Part model, mm, in its own coordinate system. Face numbers are marked on the shaded views. A direction names the side the tool comes from. Round coordinates to 2 decimals unless told otherwise and drop trailing zeros. Write each question's results on one line, items separated by ' | '. Start each with the question number.
1. Drop flat-ended pins along their axis: pin 1 Ø1 at (x, z) = (-10, -1.5) entering from +Y; pin 2 Ø14.5 at (x, y) = (5.5, 0.5) entering from +Z; pin 3 Ø0.5 at (x, z) = (-12.5, -4.5) entering from -Y; pin 4 Ø1.6 at (x, y) = (-12.5, 7.5) entering from -Z. Give the stop position or say it passes through.
2. Probe L1, parallel to Y at x = -12.5, z = -3.7 (3 decimals); L2, parallel to Y at x = 0, z = -4.05 (3 decimals); L3, parallel to Z at x = -5.25, y = 13. List the from-to ranges inside material, lowest first. Write a range as [from, to].
3. Which spindle directions (+Z, -Z, +X, -X, +Y, -Y) get a long thin tool onto all of the face, cutting with end or side? Do the marked faces 1 and 2. Say none if no direction does.
```python
from build123d import *

# Parameters (mm, degrees)
SKETCH1_R           = 15
BOSS_EXTRUDE1_DEPTH = 5
CUT_EXTRUDE1_DEPTH  = 4
FILLET1_R           = 5
FILLET2_R           = 5
SKETCH4_R           = 4.125
CUT_EXTRUDE2_DEPTH  = 22.794494718
SKETCH7_R           = 15
SKETCH7_R_2         = 12.5
CUT_EXTRUDE3_DEPTH  = 22.794494741
BOSS_EXTRUDE4_START = -2
SKETCH10_R          = 1.025
BOSS_EXTRUDE4_DEPTH = 2
FILLET5_R           = 1.5
BOSS_EXTRUDE5_START = -2
BOSS_EXTRUDE5_DEPTH = 2
FILLET6_R           = 3.125
FILLET7_R           = 0.5


with BuildPart() as part:
    # Sketch1 → Boss-Extrude1 (new body)
    with BuildSketch(Plane.XY):
        Circle(SKETCH1_R)
    extrude(amount=-BOSS_EXTRUDE1_DEPTH)

    # Sketch3 → Cut-Extrude1 (cut)
    with BuildSketch(Plane.XY):
        Polygon((8.5, 0), (0, 14.875), (-8.5, 0), (0, -14.875), align=None)
    extrude(amount=-CUT_EXTRUDE1_DEPTH, mode=Mode.SUBTRACT)

    # Fillet1
    fillet1_edges = [part.edges().sort_by_distance(p)[0] for p in [
        (0, 14.875, -2),
        (8.5, 0, -2),
        (0, -14.875, -2),
        (-8.5, 0, -2),
    ]]
    fillet(fillet1_edges, radius=FILLET1_R)

    # Fillet2
    # the kernel refuses this fillet: 5 mm, written as the material it adds along each edge
    with BuildSketch(Plane(origin=(0, -4.797177815, -4), x_dir=(-0.8682431421244594, -0.4961389383568335, 0), z_dir=(-0.4961389383568335, 0.8682431421244594, 0))) as fillet2_piece_1:
        with BuildLine():
            CenterArc((0.101020514, 5), FILLET2_R, 270, 78.463040967)
            Line((0.101020514, 0), (0.101020514, -0.1))
            Line((0.101020514, -0.1), (5, -0.1))
            Line((5, -0.1), (5.1, 0))
            ThreePointArc((5.1, 0), (5.1, 2), (5.09797959, 3.98))
            Line((5.09797959, 3.98), (5, 4))
        make_face()
    revolve(axis=Axis((0, -4.797177815, -4), (0, 0, 1)), revolution_arc=120.510237406)
    with BuildSketch(Plane(origin=(-7.082460176, -2.480694692, -4), x_dir=(1.3436192329677e-12, 7.677824188386856e-13, 1.0), z_dir=(0.49613893835683387, -0.8682431421244593, 0)), Plane(origin=(-4.341215711, 7.277872506, -4), x_dir=(1.3880008253859177e-12, -7.93143328791953e-13, 1.0), z_dir=(-0.49613893835683387, -0.8682431421244591, 0)), Plane(origin=(7.082460176, 2.480694692, -4), x_dir=(-1.3700903659455922e-12, -7.829087805403382e-13, 1.0), z_dir=(-0.49613893835683376, 0.8682431421244593, 0)), Plane(origin=(4.341215711, -7.277872506, -4), x_dir=(-1.3859204382413136e-12, 7.919545361378934e-13, 1.0), z_dir=(0.49613893835683387, 0.8682431421244593, 0))) as fillet2_piece_2:
        with BuildLine():
            CenterArc((5, -4.898979486), FILLET2_R, 101.536959033, 78.463040967)
            Line((0, -4.898979486), (-0.1, -4.898979486))
            Line((-0.1, -4.898979486), (-0.1, 0))
            Line((-0.1, 0), (0, 0.1))
            ThreePointArc((0, 0.1), (2, 0.1), (3.98, 0.09797959))
            Line((3.98, 0.09797959), (4, 0))
        make_face()
    extrude(amount=5.525154858)
    with BuildSketch(Plane(origin=(-2.741244466, 0, -4), x_dir=(-0.8682431421244594, 0.4961389383568336, 0), z_dir=(0.4961389383568336, 0.8682431421244594, 0))) as fillet2_piece_3:
        with BuildLine():
            CenterArc((0.101020514, 5), FILLET2_R, 270, 78.463040967)
            Line((0.101020514, 0), (0.101020514, -0.1))
            Line((0.101020514, -0.1), (5, -0.1))
            Line((5, -0.1), (5.1, 0))
            ThreePointArc((5.1, 0), (5.1, 2), (5.09797959, 3.98))
            Line((5.09797959, 3.98), (5, 4))
        make_face()
    revolve(axis=Axis((-2.741244466, 0, -4), (0, 0, 1)), revolution_arc=59.489762594)
    with BuildSketch(Plane(origin=(0, 4.797177815, -4), x_dir=(0.8682431421244594, 0.4961389383568332, 0), z_dir=(0.4961389383568332, -0.8682431421244594, 0))) as fillet2_piece_4:
        with BuildLine():
            CenterArc((0.101020514, 5), FILLET2_R, 270, 78.463040967)
            Line((0.101020514, 0), (0.101020514, -0.1))
            Line((0.101020514, -0.1), (5, -0.1))
            Line((5, -0.1), (5.1, 0))
            ThreePointArc((5.1, 0), (5.1, 2), (5.09797959, 3.98))
            Line((5.09797959, 3.98), (5, 4))
        make_face()
    revolve(axis=Axis((0, 4.797177815, -4), (0, 0, 1)), revolution_arc=120.510237406)
    with BuildSketch(Plane(origin=(2.741244466, 0, -4), x_dir=(0.8682431421244592, 0.49613893835683376, 0), z_dir=(-0.49613893835683376, 0.8682431421244592, 0))) as fillet2_piece_5:
        with BuildLine():
            CenterArc((0.101020514, -5), FILLET2_R, 11.536959033, 78.463040967)
            Line((0.101020514, 0), (0.101020514, 0.1))
            Line((0.101020514, 0.1), (5, 0.1))
            Line((5, 0.1), (5.1, 0))
            ThreePointArc((5.1, 0), (5.1, -2), (5.09797959, -3.98))
            Line((5.09797959, -3.98), (5, -4))
        make_face()
    revolve(axis=Axis((2.741244466, 0, -4), (0, 0, -1)), revolution_arc=59.489762594)

    # Sketch4 → Cut-Extrude2 (cut, through all)
    with BuildSketch(Plane.XY):
        Circle(SKETCH4_R)
    extrude(amount=-CUT_EXTRUDE2_DEPTH, mode=Mode.SUBTRACT)

    # Sketch7 → Cut-Extrude3 (cut, through all)
    with BuildSketch(Plane.XY):
        Circle(SKETCH7_R)
        Circle(SKETCH7_R_2, mode=Mode.SUBTRACT)
    extrude(amount=-CUT_EXTRUDE3_DEPTH, mode=Mode.SUBTRACT)

    # Sketch10 → Boss-Extrude4 (add)
    # profile 1 of 2: a face of its own
    with BuildSketch(Plane(origin=(0, 0, -5), x_dir=(-1, 0, 0), z_dir=(0, 0, -1)).offset(BOSS_EXTRUDE4_START)):
        with BuildLine():
            Line((15, 10), (7.5, 10))
            ThreePointArc((7.5, 10), (11.180339887, 5.590169944), (12.5, 0))
            ThreePointArc((12.5, 0), (11.180339887, -5.590169944), (7.5, -10))
            Line((7.5, -10), (15, -10))
            Line((15, -10), (15, 10))
        make_face()
        with Locations((12.5, -7.5)):
            Circle(SKETCH10_R, mode=Mode.SUBTRACT)
        with Locations((12.5, 7.5)):
            Circle(SKETCH10_R, mode=Mode.SUBTRACT)
    # profile 2 of 2: a face of its own
    with BuildSketch(Plane(origin=(0, 0, -5), x_dir=(-1, 0, 0), z_dir=(0, 0, -1)).offset(BOSS_EXTRUDE4_START)):
        with BuildLine():
            Line((-7.5, 10), (-15, 10))
            Line((-15, 10), (-15, -10))
            Line((-15, -10), (-7.5, -10))
            ThreePointArc((-7.5, -10), (-12.5, 0), (-7.5, 10))
        make_face()
        with Locations((-12.5, -7.5)):
            Circle(SKETCH10_R, mode=Mode.SUBTRACT)
        with Locations((-12.5, 7.5)):
            Circle(SKETCH10_R, mode=Mode.SUBTRACT)
    extrude(amount=BOSS_EXTRUDE4_DEPTH)

    # Fillet5
    fillet5_edges = [part.edges().sort_by_distance(p)[0] for p in [
        (15, -10, -4),
        (15, 10, -4),
        (-15, 10, -4),
        (-15, -10, -4),
    ]]
    fillet(fillet5_edges, radius=FILLET5_R)

    # Sketch11 → Boss-Extrude5 (add)
    with BuildSketch(Plane(origin=(0, 0, -5), x_dir=(-1, 0, 0), z_dir=(0, 0, -1)).offset(BOSS_EXTRUDE5_START)):
        with BuildLine():
            ThreePointArc((-7.5, 10), (0, 12.5), (7.5, 10))
            Line((7.5, 10), (10.5, 10))
            ThreePointArc((10.5, 10), (0, 14.5), (-10.5, 10))
            Line((-10.5, 10), (-7.5, 10))
        make_face()
        with BuildLine():
            Line((10.5, -10), (7.5, -10))
            ThreePointArc((7.5, -10), (0, -12.5), (-7.5, -10))
            Line((-7.5, -10), (-10.5, -10))
            ThreePointArc((-10.5, -10), (0, -14.5), (10.5, -10))
        make_face()
    extrude(amount=BOSS_EXTRUDE5_DEPTH)

    # Fillet6
    fillet6_edges = [part.edges().sort_by_distance(p)[0] for p in [
        (-10.5, 10, -4),
        (10.5, 10, -4),
        (10.5, -10, -4),
        (-10.5, -10, -4),
    ]]
    fillet(fillet6_edges, radius=FILLET6_R)

    # Fillet7
    fillet7_edges = [part.edges().sort_by_distance(p)[0] for p in [
        (5.711837943, 4.879283599, 0),
        (5.711837943, -4.879283599, 0),
        (-5.711837943, -4.879283599, 0),
        (-5.711837943, 4.879283599, 0),
        (7.741244466, 0, 0),
        (0, -9.797177815, 0),
        (-7.741244466, 0, 0),
        (0, 9.797177815, 0),
    ]]
    fillet(fillet7_edges, radius=FILLET7_R)


solid = part.part
```
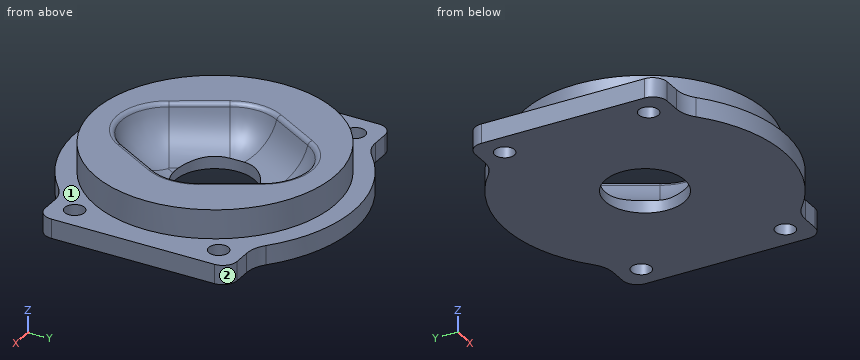
Solution:
1) pin 1: y = 8.12 | pin 2: z = 0 | pin 3: y = -10 | pin 4: through
2) L1: [-10, -8.525], [-6.475, 6.475], [8.525, 10] | L2: [-14.5, -4.125], [4.125, 14.5] | L3: [-5, -3]
3) face 1: +Z | face 2: +Z, -Z, +X, +Y
